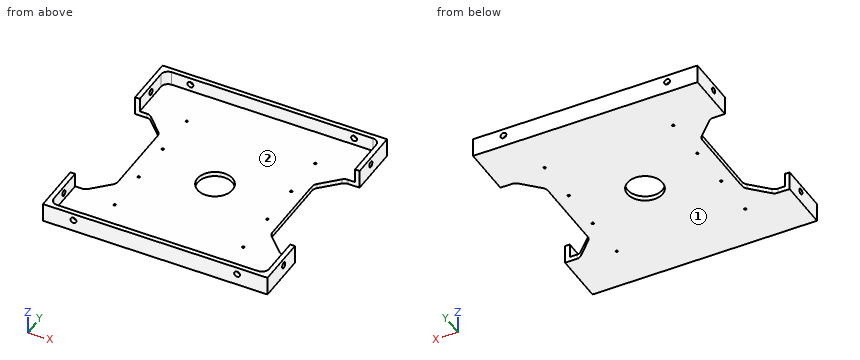
```python
from build123d import *

# Parameters (mm, degrees)
SKETCH1_W                       = 96
SKETCH1_H                       = 96
BOSS_EXTRUDE1_DEPTH             = 8
SKETCH2_W                       = 92
SKETCH2_H                       = 92
COMPONENT_PLATFORM_DEPTH        = 6
CABLE_SLOTS_DEPTH               = 6
SKETCH4_R                       = 7.5
CENTER_MASS_CUT_DEPTH           = 6
INNER_CORNER_FILLETS_R          = 3
TAP_DRILL_FOR_M3X0_5_TAP4_D     = 2.5
TAP_DRILL_FOR_M3X0_5_TAP4_DEPTH = 2
TAP_DRILL_FOR_M1_2X0_25_TAP1_D  = 0.95
TAP_DRILL_FOR_M3X0_5_TAP3_D     = 2.5
TAP_DRILL_FOR_M3X0_5_TAP3_DEPTH = 2


with BuildPart() as part:
    # Sketch1 → Boss-Extrude1 (new body)
    with BuildSketch(Plane.XY):
        Rectangle(SKETCH1_W, SKETCH1_H)
    extrude(amount=BOSS_EXTRUDE1_DEPTH)

    # Sketch2 → Component Platform (cut)
    with BuildSketch(Plane.XY.offset(8)):
        Rectangle(SKETCH2_W, SKETCH2_H)
    extrude(amount=-COMPONENT_PLATFORM_DEPTH, mode=Mode.SUBTRACT)

    # Sketch3 → Cable Slots (cut, symmetric)
    with BuildSketch(Plane.XY.offset(2)):
        with BuildLine():
            Line((-40.878679656, -25.121320344), (-33.878679656, -18.121320344))
            ThreePointArc((-33.878679656, -18.121320344), (-33.228361402, -17.148050297), (-33, -16))
            Line((-33, -16), (-33, 16))
            ThreePointArc((-33, 16), (-33.228361402, 17.148050297), (-33.878679656, 18.121320344))
            Line((-33.878679656, 18.121320344), (-40.878679656, 25.121320344))
            ThreePointArc((-40.878679656, 25.121320344), (-41.851949703, 25.771638598), (-43, 26))
            Line((-43, 26), (-48, 26))
            Line((-48, 26), (-48, -26))
            Line((-48, -26), (-43, -26))
            ThreePointArc((-43, -26), (-41.851949703, -25.771638598), (-40.878679656, -25.121320344))
        make_face()
        with BuildLine():
            Line((48, -26), (48, 26))
            Line((48, 26), (43, 26))
            ThreePointArc((43, 26), (41.851949703, 25.771638598), (40.878679656, 25.121320344))
            Line((40.878679656, 25.121320344), (33.878679656, 18.121320344))
            ThreePointArc((33.878679656, 18.121320344), (33.228361402, 17.148050297), (33, 16))
            Line((33, 16), (33, -16))
            ThreePointArc((33, -16), (33.228361402, -17.148050297), (33.878679656, -18.121320344))
            Line((33.878679656, -18.121320344), (40.878679656, -25.121320344))
            ThreePointArc((40.878679656, -25.121320344), (41.851949703, -25.771638598), (43, -26))
            Line((43, -26), (48, -26))
        make_face()
    extrude(amount=CABLE_SLOTS_DEPTH, both=True, mode=Mode.SUBTRACT)

    # Sketch4 → Center Mass Cut (cut)
    with BuildSketch(Plane.XY.offset(2)):
        Circle(SKETCH4_R)
    extrude(amount=-CENTER_MASS_CUT_DEPTH, mode=Mode.SUBTRACT)

    # Inner Corner Fillets
    inner_corner_fillets_edges = [part.edges().sort_by_distance(p)[0] for p in [
        (-46, -46, 5),
        (-46, 46, 5),
        (46, 46, 5),
        (46, -46, 5),
    ]]
    fillet(inner_corner_fillets_edges, radius=INNER_CORNER_FILLETS_R)

    # Tap Drill for M3x0.5 Tap4
    with Locations(Plane(origin=(0, -48, 0), x_dir=(-1, 0, 0), z_dir=(0, -1, 0))):
        with Locations((35, -5), (-35, -5)):
            tap_drill_for_m3x0_5_tap4 = Hole(TAP_DRILL_FOR_M3X0_5_TAP4_D / 2, depth=TAP_DRILL_FOR_M3X0_5_TAP4_DEPTH)

    # Mirror2: Tap Drill for M3x0.5 Tap4 across plane
    add(tap_drill_for_m3x0_5_tap4.mirror(Plane(origin=(0, 0, 0), x_dir=(0, 0, 1), z_dir=(0, -1, 0))), mode=Mode.SUBTRACT)

    # Tap Drill for M1.2x0.25 Tap1 (through all)
    with Locations(Plane.XY.offset(2)):
        with Locations((-27.5, 28.95), (-27.5, 9.65), (-27.5, -9.65), (-27.5, -28.95), (27.5, -28.95), (27.5, -9.65), (27.5, 9.65), (27.5, 28.95)):
            Hole(TAP_DRILL_FOR_M1_2X0_25_TAP1_D / 2)

    # Tap Drill for M3x0.5 Tap3
    with Locations(Plane(origin=(48, 0, 0), x_dir=(0, 0, -1), z_dir=(1, 0, 0))):
        with Locations((-5, -35), (-5, 35)):
            tap_drill_for_m3x0_5_tap3 = Hole(TAP_DRILL_FOR_M3X0_5_TAP3_D / 2, depth=TAP_DRILL_FOR_M3X0_5_TAP3_DEPTH)

    # Mirror3: Tap Drill for M3x0.5 Tap3 across plane
    add(tap_drill_for_m3x0_5_tap3.mirror(Plane(origin=(0, 0, 0), x_dir=(0, 0, 1), z_dir=(1, 0, 0))), mode=Mode.SUBTRACT)


solid = part.part
```
For this review, take the finished solid that the model builds, in its own axes (mm). Face numbers are marked on the shaded views. Give positions to 0.01 mm unless a question says otherwise; leave off trailing zeros. Write each loop counter-clockwise with the first axis right and the second up, starting at its lowest first coordinate (ties: lowest second). Pieces come first, ordered by that corner, then holes. Notation, with made-up numbers: M 67.25,-11 L 86.25,-11 A23 cw 86.25,-1 Z; hole C -22.75,-19.75 d3. An arc over 180 degrees is marked long. One line per item, written item: value.
1) For line 1 (Y direction, x = -27.5, z = 1.25) (3 decimals); line 2 (X direction, y = 46.4, z = 5); line 3 (X direction, y = 28, z = 7.5), list the stretches that pass through material, from the lowest coordinate up. Write a range as from..to.
Results are:
line 1: y = -48..-29.425, -28.475..-10.125, -9.175..9.175, 10.125..28.475, 29.425..48
line 2: x = -48..-36.25, -33.75..33.75, 36.25..48
line 3: x = -48..-46, 46..48
2) Take a section at A-A, the plane y = 0. Write out the cut boundary in (x, z).
Results are:
outline: M -33,0 L -7.5,0 L -7.5,2 L -33,2 Z; M 7.5,0 L 33,0 L 33,2 L 7.5,2 Z
3) Take a section at D-D, the plane y = -32.5. Write out the cut boundary in (x, z).
Results are:
outline: M -48,0 L 48,0 L 48,8 L 46,8 L 46,2 L -46,2 L -46,8 L -48,8 Z
4) The part is to be moulded in two halves that separate along Y. For the marked faces 1 and 2, say which applies: +Y half, -Y half, draft (parallel to the pull), parting line (faces both ways), or undercut.
Results are:
face 1: draft
face 2: undercut
5) Take a section at B-B, the plane x = -35. Write out the cut boundary in (y, z), then the cut area to 3 significant figures.
Results are:
outline: M -48,0 L -19.24,0 L -19.24,2 L -46,2 L -46,3.75 L -48,3.75 Z; M -48,6.25 L -46,6.25 L -46,8 L -48,8 Z; M 19.24,0 L 48,0 L 48,3.75 L 46,3.75 L 46,2 L 19.24,2 Z; M 46,6.25 L 48,6.25 L 48,8 L 46,8 Z
area: 129 mm²
6) Take a section at C-C, the plane y = 35. Write out the cut boundary in (x, z).
Results are:
outline: M -48,0 L 48,0 L 48,3.75 L 46,3.75 L 46,2 L -46,2 L -46,3.75 L -48,3.75 Z; M -48,6.25 L -46,6.25 L -46,8 L -48,8 Z; M 46,6.25 L 48,6.25 L 48,8 L 46,8 Z
